from build123d import *

# Parameters (mm, degrees)
F1_DEPTH       = 8
F1_DEPTH_BACK  = 8
F3_D           = 6
F3_START       = 12.7000001
F3_CBORE_D     = 10
F3_CBORE_DEPTH = 17.3
F4_R           = 0.5


with BuildPart() as f1:
    # F0 (on Right) → F1 (new body, two sides)
    with BuildSketch(Plane.YZ) as f1_sk:
        with BuildLine():
            Line((-19, -29), (-19, -36))
            Line((-19, -36), (19, -36))
            Line((19, -36), (19, -27.7320508076))
            ThreePointArc((19, -27.7320508076), (22, -26), (19, -24.2679491924))
            Line((19, -24.2679491924), (19, -16.2))
            Line((19, -16.2), (19, 8))
            ThreePointArc((19, 8), (13.8227400876, 12.0330174031), (11.1791699801, 6.026288954))
            ThreePointArc((11.1791699801, 6.026288954), (0, -12.7), (-11.1791699801, 6.026288954))
            ThreePointArc((-11.1791699801, 6.026288954), (-13.8227400876, 12.0330174031), (-19, 8))
            Line((-19, 8), (-19, -23))
            Line((-19, -23), (-21, -23))
            Line((-21, -23), (-21, -24.2679491924))
            ThreePointArc((-21, -24.2679491924), (-18, -26), (-21, -27.7320508076))
            Line((-21, -27.7320508076), (-21, -29))
            Line((-21, -29), (-19, -29))
        make_face()
    extrude(amount=F1_DEPTH)
    extrude(f1_sk.sketch, amount=-F1_DEPTH_BACK)

    # F3 (through all)
    # its depths count from where the whole tool has entered the part; down to there all is cleared
    with Locations(Plane.XY.offset(-F3_START)):
        with Locations((0, 0)):
            CounterBoreHole(F3_D / 2, F3_CBORE_D / 2, F3_CBORE_DEPTH)

    # F4
    f4_edges = [f1.edges().sort_by_distance(p)[0] for p in [
        (0, -21, -23),
        (0, -21, -29),
    ]]
    fillet(f4_edges, radius=F4_R)


solid = f1.part
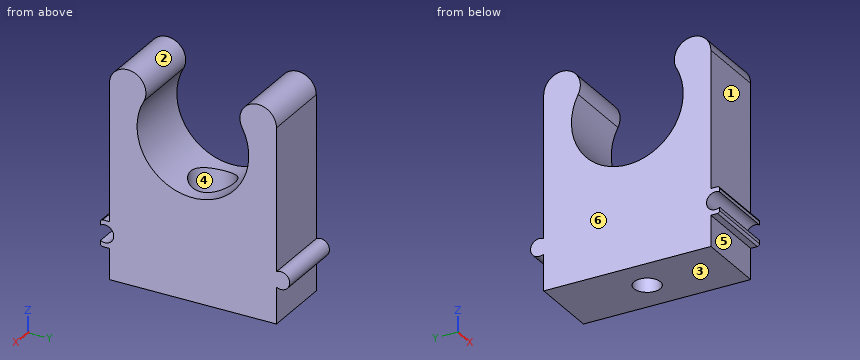
For this review, take the finished solid that the model builds, in its own axes (mm). Face numbers are marked on the shaded views. A direction names the side the tool comes from. Round coordinates to 2 decimals unless told otherwise and drop trailing zeros. Order: outer loops, then holes, each group sorted by start corner. A loop starts at its lowest first (then second) coordinate and runs counter-clockwise, first axis right, second up. Notation, with made-up numbers: (-18.5, 43.25) -> (19.5, 43.25) arc R23 ccw to (19.5, 72.25) -> close; hole circle Ø3 at (-15.5, 80.5). An arc over 180 degrees is marked (long way). Write item = value, one per line. Start each with the question number.
1) The part is to be moulded in two halves that separate along Y. For the marked faces 1, 2 and 3, say which applies: +Y half, -Y half, draft (parallel to the pull), parting line (faces both ways), or undercut.
2) Take a section at A-A on y = 0. State the section outline as (x, z) points, plus the area to 3 significant figures.
3) Tool access review of the marked faces 4, 5 and 6: name each direction out of +Z, -Z, +X, -X, +Y, -Y from which nothing blocks a thin tool from reaching the whole face with its end or side.
4) Take a section at C-C on z = -26. State the section outline as (x, y) points.
5) Take a section at D-D on x = 0.5. State the section outline as (y, z) points, plus the area to 3 significant figures.
6) Take a section at B-B on z = 0. State the section outline as (x, y) points, plus the area to 3 significant figures.
7) To check wall thickness, follow line 1 (X direction, y = 0, z = -25); line 2 (Y direction, x = -4, z = 0); line 3 (Z direction, x = -2.25, y = -20). State the ranges of each line that lie inside material, in increasing order. Write a range as from..to.
8) Insertion check: pin 1 (3.5 mm diameter, centred on x = 3, z = -34, fed in from -Y); pin 2 (1.2 mm diameter, centred on x = 3, y = -20, fed in from -Z); pin 3 (1.5 mm diameter, centred on x = 4, z = -30, fed in from +Y). Each pin has a flat end and moves straight along its axis. Give the tip position at first contact, or say it passes through.
Verdict:
q1.face_1 = -Y half
q1.face_2 = undercut
q1.face_3 = draft
q2.outline = (-8, -36) -> (-3, -36) -> (-3, -30) -> (-5, -30) -> (-5, -12.7) -> (-8, -12.7) -> close; (3, -36) -> (8, -36) -> (8, -12.7) -> (5, -12.7) -> (5, -30) -> (3, -30) -> close
q2.area = 164 mm2
q3.face_4 = +Z
q3.face_5 = -Z, +X, -X, -Y
q3.face_6 = +Z, -Z, -X, +Y, -Y
q4.outline = (-8, -18) -> (8, -18) -> (8, 22) -> (-8, 22) -> close; hole circle Ø10 at (0, 0)
q5.outline = (-21, -28.5) arc R0.5 ccw to (-20.5, -29) -> (-19, -29) -> (-19, -36) -> (-2.96, -36) -> (-2.96, -30) -> (-4.97, -30) -> (-4.97, -11.69) arc R12.7 cw to (-11.18, 6.03) arc R4.16 ccw (long way) to (-19, 8) -> (-19, -23) -> (-20.5, -23) arc R0.5 ccw to (-21, -23.5) -> (-21, -24.27) arc R2 cw (long way) to (-21, -27.73) -> close; (2.96, -36) -> (19, -36) -> (19, -27.73) arc R2 ccw (long way) to (19, -24.27) -> (19, 8) arc R4.16 ccw (long way) to (11.18, 6.03) arc R12.7 cw to (4.97, -11.69) -> (4.97, -30) -> (2.96, -30) -> close
q5.area = 1,080 mm2
q6.outline = (-8, -19) -> (8, -19) -> (8, -12.7) -> (-8, -12.7) -> close; (-8, 12.7) -> (8, 12.7) -> (8, 19) -> (-8, 19) -> close
q6.area = 202 mm2
q7.line_1 = -8..-5, 5..8
q7.line_2 = -19..-12.7, 12.7..19
q7.line_3 = -29..-28, -24..-23
q8.pin_1 = -19
q8.pin_2 = -29
q8.pin_3 = 19
